from build123d import *

# Parameters (mm, degrees)
BOSS_EXTRUDE1_DEPTH   = 7
SKETCH2_R             = 19
CUT_EXTRUDE1_DEPTH    = 5
SKETCH3_R             = 6
SKETCH3_R_2           = 1.6
CUT_EXTRUDE2_DEPTH    = 5
M3_TAPPED_HOLE1_D     = 2.5
M3_TAPPED_HOLE1_DEPTH = 5
M3_TAPPED_HOLE1_TIP   = 0.751075774
SKETCH6_R             = 1.5
CUT_EXTRUDE3_DEPTH    = 7


with BuildPart() as part:
    # Sketch1 → Boss-Extrude1 (new body)
    with BuildSketch(Plane.XY):
        with BuildLine():
            Line((31, 3.5), (21, 3.5))
            Line((21, 3.5), (21, 20.5))
            ThreePointArc((21, 20.5), (0, 41.5), (-21, 20.5))
            Line((-21, 20.5), (-21, 3.5))
            Line((-21, 3.5), (-31, 3.5))
            Line((-31, 3.5), (-31, -3.5))
            Line((-31, -3.5), (31, -3.5))
            Line((31, -3.5), (31, 3.5))
        make_face()
    extrude(amount=BOSS_EXTRUDE1_DEPTH)

    # Sketch2 → Cut-Extrude1 (cut)
    with BuildSketch(Plane.XY.offset(7)):
        with Locations((0, 20.5)):
            Circle(SKETCH2_R)
    extrude(amount=-CUT_EXTRUDE1_DEPTH, mode=Mode.SUBTRACT)

    # Sketch3 → Cut-Extrude2 (cut)
    with BuildSketch(Plane.XY.offset(2)):
        with Locations((0, 13.5)):
            Circle(SKETCH3_R)
        with Locations((15.5, 20.5)):
            Circle(SKETCH3_R_2)
        with Locations((-15.5, 20.5)):
            Circle(SKETCH3_R_2)
    extrude(amount=-CUT_EXTRUDE2_DEPTH, mode=Mode.SUBTRACT)

    # M3 Tapped Hole1
    with Locations(Plane(origin=(-14, -3.5, 3.5), x_dir=(0, 0, -1), z_dir=(0, -1, 0))):
        with Locations((0, 0), (0, 28)):
            Hole(M3_TAPPED_HOLE1_D / 2, depth=M3_TAPPED_HOLE1_DEPTH)
            with Locations((0, 0, -(M3_TAPPED_HOLE1_DEPTH + M3_TAPPED_HOLE1_TIP / 2))):  # 118° drill point
                Cone(0, M3_TAPPED_HOLE1_D / 2, M3_TAPPED_HOLE1_TIP, mode=Mode.SUBTRACT)

    # Sketch6 → Cut-Extrude3 (cut)
    with BuildSketch(Plane(origin=(0, 3.5, 0), x_dir=(1, 0, 0), z_dir=(0, 1, 0))):
        with Locations(Location((-26, -3.5, 0), (0, 0, 270))):
            Circle(SKETCH6_R)
        with Locations(Location((26, -3.5, 0), (0, 0, 270))):
            Circle(SKETCH6_R)
    extrude(amount=-CUT_EXTRUDE3_DEPTH, mode=Mode.SUBTRACT)


solid = part.part
Check sheet for the modelled part. Datum: model origin and axes. Units: mm. A direction names the side the tool comes from. Round coordinates to 2 decimals unless told otherwise and drop trailing zeros. Order: outer loops, then holes, each group sorted by start corner. A loop starts at its lowest first (then second) coordinate and runs counter-clockwise, first axis right, second up. Notation, with made-up numbers: M 17,1.5 L 39,1.5 A21 cw 39,26.5 Z; hole C 60,15.25 d9. An arc over 180 degrees is marked long. One line per item, written item: value. Start each with the question number.
1. Access from +Z, -Z, +X, -X, +Y, -Y to the whole of each face (thin tool, end or side, straight path). Record for faces 1 (the cylindrical face through (-12.946, -0.965, 4.172)), 2 (the flat face through (-25, 3.5, 5)), 3 (the flat face through (27, 3.5, 5)), 4 (the cylindrical face through (10.214, 36.521, 4.535)).
2. Scan lines: line 1 along X through (y, z) = (-0.5, 3.5); line 2 along Y through (x, z) = (0, 4.65); line 3 along Y through (x, z) = (0, 0.5). Record each from-to range of solid material in increasing order.
3. Section check D-D on x = 18. Enter the section's corners in (y, z), and give its area (3 significant figures).
4. Section check C-C on y = 30. Enter the section's corners in (x, z).
5. Section check A-A on x = -26. Enter the section's corners in (y, z).
6. Release check for a two-part mould opening along Y. For faces 5 (the flat face through (6.5, 14.3, 0)), 6 (the cylindrical face through (0.462, 41.495, 3.451)), 7 (the flat face through (0, 21, 2)) record: released by +Y, released by -Y, zero draft, split by the parting line, or undercut.
7. Section check B-B on z = 1. Enter the section's corners in (x, y), and give its area (3 significant figures).
8. Gauge pin test, flat ends, axial feed: P1, Ø4, axis at x = 9, y = 28, coming from the +Z side; P2, Ø3.5, axis at x = 26, z = 3.5, coming from the +Y side; P3, Ø1.5, axis at y = 14, z = 4.5, coming from the -X side. Record the tip position at first contact, or that the pin passes through.
Results found:
1. face 1: -Y
1. face 2: +Z, -Z, -X, +Y
1. face 3: +Z, -Z, +X, +Y
1. face 4: +Z
2. line 1: -31 to -27.5, -24.5 to -15.25, -12.75 to 12.75, 15.25 to 24.5, 27.5 to 31
2. line 2: -3.5 to 1.5, 39.5 to 41.5
2. line 3: -3.5 to 7.5, 19.5 to 41.5
3. outline: M -3.5,0 L 31.32,0 L 31.32,7 L 26.58,7 L 26.58,2 L 14.42,2 L 14.42,7 L -3.5,7 Z
3. area: 183 mm^2
4. outline: M -18.73,0 L 18.73,0 L 18.73,7 L 16.45,7 L 16.45,2 L -16.45,2 L -16.45,7 L -18.73,7 Z
5. outline: M -3.5,0 L 3.5,0 L 3.5,2 L -3.5,2 Z; M -3.5,5 L 3.5,5 L 3.5,7 L -3.5,7 Z
6. face 5: zero draft
6. face 6: released by +Y
6. face 7: undercut
7. outline: M -31,-3.5 L 31,-3.5 L 31,3.5 L 21,3.5 L 21,20.5 A21 ccw -21,20.5 L -21,3.5 L -31,3.5 Z; hole C -15.5,20.5 d3.2; hole C 0,13.5 d12; hole C 15.5,20.5 d3.2
7. area: 1,710 mm^2
8. P1: z = 2
8. P2: y = 3.5
8. P3: x = -21
